Design review of the part built by this model. Coordinates are the model's own, in mm. Face numbers are marked on the shaded views. A direction names the side the tool comes from. Give positions to 0.01 mm unless a question says otherwise; leave off trailing zeros. Order: outer loops, then holes, each group sorted by start corner. A loop starts at its lowest first (then second) coordinate and runs counter-clockwise, first axis right, second up. Notation, with made-up numbers: (75, -6) -> (117, -6) arc R17 ccw to (117, 13) -> close; hole circle Ø2 at (-14, 72.25). An arc over 180 degrees is marked (long way). One line per item, written item: value. Start each with the question number.
1) Consider section A-A (x = -14.75). State the section outline as (y, z) points.
2) Consider section D-D (y = -9). State the section outline as (x, z) points, plus the area to 3 significant figures.
3) The part is to be moulded in two halves that separate along Z. For the marked faces 6, 7 and 8, say which applies: released by +Z, released by -Z, zero draft, split by the parting line, or undercut.
4) Tool access review of the marked faces 1, 2, 3, 4 and 5: name each direction out of +Z, -Z, +X, -X, +Y, -Y from which nothing blocks a thin tool from reaching the whole face with its end or side.
5) Wall thickness on line 1 along Y through (x, z) = (-14.75, -14.3); line 2 along X through (y, z) = (0.75, -31); line 3 along Z through (x, y) = (4, -5.25): over which ranges is each line inside the solid? List them lowest first. Write a range as from..to.
6) Consider section C-C (x = 34.75). State the section outline as (y, z) points.
7) Consider section B-B (y = -5). State the section outline as (x, z) points, plus the area to 3 significant figures.
8) For pin 1 (2 mm diameter, centred on y = -5.5, z = -37, fed in from +X); pin 2 (6.5 mm diameter, centred on x = -23.5, y = -0.5, fed in from +Z); pin 3 (4 mm diameter, centred on y = 0.5, z = -12.5, fed in from -X); pin 4 (3.5 mm diameter, centred on x = 34.75, y = -5, fed in from +Z), all flat-tipped, find the tip position at first contact; note any pin that passes through.
from build123d import *

# Parameters (mm, degrees)
SKETCH1_R           = 3
BOSS_EXTRUDE1_DEPTH = 2.5
SKETCH2_W           = 40
SKETCH2_H           = 20
BOSS_EXTRUDE2_DEPTH = 41.5
BOSS_EXTRUDE3_START = -27.8
SKETCH3_W           = 7.25
SKETCH3_H           = 20
BOSS_EXTRUDE3_DEPTH = 3
SKETCH4_R           = 2
CUT_EXTRUDE1_DEPTH  = 50.357902103
SKETCH5_W           = 3
SKETCH5_H           = 8
BOSS_EXTRUDE4_DEPTH = 20


with BuildPart() as part:
    # Sketch1 → Boss-Extrude1 (new, symmetric)
    with BuildSketch(Plane.XY):
        Circle(SKETCH1_R)
    extrude(amount=BOSS_EXTRUDE1_DEPTH, both=True)

    # Sketch2 → Boss-Extrude2 (add)
    with BuildSketch(Plane(origin=(0, 0, -2.5), x_dir=(-1, 0, 0), z_dir=(0, 0, -1))):
        with Locations((-10, 0)):
            Rectangle(SKETCH2_W, SKETCH2_H)
    extrude(amount=BOSS_EXTRUDE2_DEPTH)

    # Sketch3 → Boss-Extrude3 (add)
    with BuildSketch(Plane(origin=(0, 0, -44), x_dir=(-1, 0, 0), z_dir=(0, 0, -1)).offset(BOSS_EXTRUDE3_START)):
        with Locations((-33.625, 0)):
            Rectangle(SKETCH3_W, SKETCH3_H)
        with Locations((13.625, 0)):
            Rectangle(SKETCH3_W, SKETCH3_H)
    extrude(amount=-BOSS_EXTRUDE3_DEPTH)

    # Sketch4 → Cut-Extrude1 (cut, through all)
    with BuildSketch(Plane.XY.offset(-13.2)):
        with Locations((-14.75, -5)):
            Circle(SKETCH4_R)
        with Locations((-14.75, 5)):
            Circle(SKETCH4_R)
        with Locations((34.75, 5)):
            Circle(SKETCH4_R)
        with Locations((34.75, -5)):
            Circle(SKETCH4_R)
    extrude(amount=-CUT_EXTRUDE1_DEPTH, mode=Mode.SUBTRACT)

    # Sketch5 → Boss-Extrude4 (add)
    with BuildSketch(Plane.ZY.offset(10)):
        with Locations((-42.5, 0)):
            Rectangle(SKETCH5_W, SKETCH5_H)
    extrude(amount=BOSS_EXTRUDE4_DEPTH)


solid = part.part
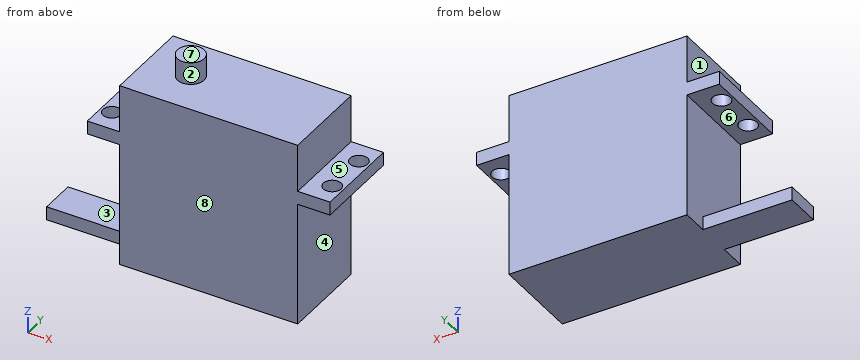
Checked values:
1. outline: (-10, -16.2) -> (-7, -16.2) -> (-7, -13.2) -> (-10, -13.2) -> close; (-4, -44) -> (4, -44) -> (4, -41) -> (-4, -41) -> close; (-3, -16.2) -> (3, -16.2) -> (3, -13.2) -> (-3, -13.2) -> close; (7, -16.2) -> (10, -16.2) -> (10, -13.2) -> (7, -13.2) -> close
2. outline: (-17.25, -16.2) -> (-10, -16.2) -> (-10, -44) -> (30, -44) -> (30, -16.2) -> (37.25, -16.2) -> (37.25, -13.2) -> (30, -13.2) -> (30, -2.5) -> (-10, -2.5) -> (-10, -13.2) -> (-17.25, -13.2) -> close
2. area: 1,700 mm^2
3. face 6: undercut
3. face 7: released by +Z
3. face 8: zero draft
4. face 1: +Z, -X, +Y, -Y
4. face 2: +Z
4. face 3: -X, +Y, -Y
4. face 4: -Z, +X, +Y, -Y
4. face 5: +Z, +X, +Y, -Y
5. line 1: y = -10..-7, -3..3, 7..10
5. line 2: x = -10..30
5. line 3: z = -44..-2.5
6. outline: (-10, -16.2) -> (-7, -16.2) -> (-7, -13.2) -> (-10, -13.2) -> close; (-3, -16.2) -> (3, -16.2) -> (3, -13.2) -> (-3, -13.2) -> close; (7, -16.2) -> (10, -16.2) -> (10, -13.2) -> (7, -13.2) -> close
7. outline: (-17.25, -16.2) -> (-16.75, -16.2) -> (-16.75, -13.2) -> (-17.25, -13.2) -> close; (-12.75, -16.2) -> (-10, -16.2) -> (-10, -44) -> (30, -44) -> (30, -16.2) -> (32.75, -16.2) -> (32.75, -13.2) -> (30, -13.2) -> (30, -2.5) -> (-10, -2.5) -> (-10, -13.2) -> (-12.75, -13.2) -> close; (36.75, -16.2) -> (37.25, -16.2) -> (37.25, -13.2) -> (36.75, -13.2) -> close
7. area: 1,680 mm^2
8. pin 1: stops at x = 30
8. pin 2: stops at z = -41
8. pin 3: stops at x = -17.25
8. pin 4: passes through
